The listing builds one solid part. Answer for the finished solid, in the listing's coordinates (mm). Give positions to 0.01 mm unless a question says otherwise; leave off trailing zeros. Loops run counter-clockwise (first coordinate to the right, second up) from the corner with the lowest first, then second, coordinate; pieces in that order, holes last.
Item 1: Each of these flat-tipped pins is pushed along its axis until it touches: pin 1 Ø8 at (x, z) = (-3, 14.5) entering from +Y; pin 2 Ø0.9 at (x, y) = (-12, -1.5) entering from -Z; pin 3 Ø1.5 at (y, z) = (-2, -2) entering from -X; pin 4 Ø0.9 at (y, z) = (-1, -1) entering from +X. Where does it stop, or does it pass through?
Item 2: Section C-C, the plane x = 0.5 is taken. Give the vertices of the cut face in (y, z).
Item 3: Section A-A, the plane y = -1.15 is taken. Give the vertices of the cut face in (x, z), and give its area (3 significant figures).
Item 4: Section B-B, the plane z = 35 is taken. Give the vertices of the cut face in (x, y), and give its area (3 significant figures).
Item 5: Consider line 1 along X through (y, z) = (-1.95, 35); line 2 along X through (y, z) = (-1.8, 29.5); line 3 along Z through (x, y) = (6, -2.3). Determine where each line is inside the solid, lowest interval first.
Item 6: Section D-D, the plane x = -8 is taken. Give the vertices of the cut face in (y, z), and give its area (3 significant figures).
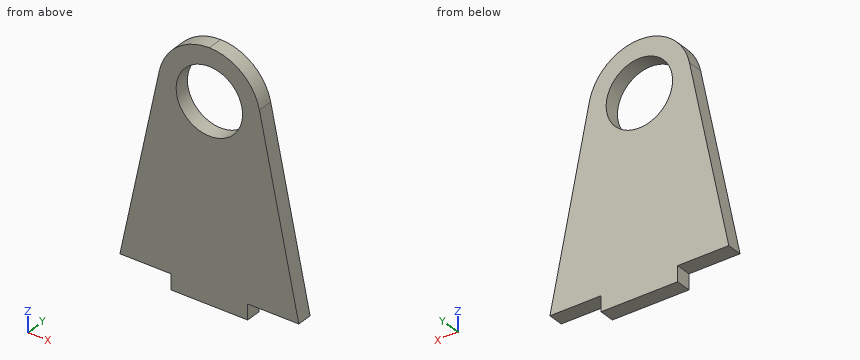
from build123d import *

# Parameters (mm, degrees)
F1_DEPTH = 3


with BuildPart() as f1:
    # F0 (on Front) → F1 (new body)
    with BuildSketch(Plane.XZ):
        with BuildLine():
            ThreePointArc((0, 45), (-6.309545, 42.758198), (-9.790141, 37.037927))
            Line((-9.790141, 37.037927), (-17.5, 0))
            Line((-17.5, 0), (-7.5, 0))
            Line((-7.5, 0), (-7.5, -3))
            Line((-7.5, -3), (0, -3))
            Line((0, -3), (7.5, -3))
            Line((7.5, -3), (7.5, 0))
            Line((7.5, 0), (17.5, 0))
            Line((17.5, 0), (9.790141, 37.037927))
            ThreePointArc((9.790141, 37.037927), (6.309545, 42.758198), (0, 45))
        make_face()
        with BuildLine():
            ThreePointArc((0, 28.5), (-6.5, 35), (0, 41.5))
            ThreePointArc((0, 41.5), (6.5, 35), (0, 28.5))
        make_face(mode=Mode.SUBTRACT)
    extrude(amount=F1_DEPTH)


solid = f1.part
Worked answers:
1. pin 1: stops at y = 0
1. pin 2: stops at z = 0
1. pin 3: stops at x = -7.5
1. pin 4: stops at x = 7.5
2. outline: (-3, -3) - (0, -3) - (0, 28.52) - (-3, 28.52) - close; (-3, 41.48) - (0, 41.48) - (0, 44.99) - (-3, 44.99) - close
3. outline: (-17.5, 0) - (-7.5, 0) - (-7.5, -3) - (7.5, -3) - (7.5, 0) - (17.5, 0) - (9.79, 37.04) arc R10 ccw to (0, 45) arc R10 ccw to (-9.79, 37.04) - close; hole circle Ø13 at (0, 35)
3. area: 1,040 mm2
4. outline: (-10.21, -3) - (-6.5, -3) - (-6.5, 0) - (-10.21, 0) - close; (6.5, -3) - (10.21, -3) - (10.21, 0) - (6.5, 0) - close
4. area: 22.3 mm2
5. line 1: x = -10.21 to -6.5, 6.5 to 10.21
5. line 2: x = -11.36 to -3.46, 3.46 to 11.36
5. line 3: z = -3 to 32.5, 37.5 to 43
6. outline: (-3, 0) - (0, 0) - (0, 41) - (-3, 41) - close
6. area: 123 mm2
